Study the drawing (mm; zero at the part's minimum x, y, z) and answer. Coordinates: 2 decimals unless noted, no trailing zeros. Write each loop counter-clockwise with the first axis right and the second up, starting at its lowest first coordinate (ties: lowest second). Pieces come first, ordered by that corner, then holes. Notation, with made-up numbers: (-33, 66.5) -> (-9, 66.5) arc R17 cw to (-9, 93.5) -> close; hole circle Ø10 at (50.5, -9). An arc over 180 degrees is marked (long way). Write item = value, one per line. Start each with the question number.
1) Flat-ended cylindrical pins translate along their axes: pin 1 Ø8 at (y, z) = (230.5, 94.5) entering from +X; pin 2 Ø5 at (x, y) = (8, 4) entering from -Z; pin 3 Ø6.5 at (x, z) = (14.5, 8.5) entering from +Y. Find the tip coordinate at first contact, or state that the pin passes through.
2) Section C-C (x = 8.5) is taken. Determine the outline of the cut face in (y, z) (1 decimal).
3) For a pull along Z with two mould halves and no side action, classify the marked faces 1, 2, 3 and 4 as released by +Z, released by -Z, zero draft, split by the parting line, or undercut.
4) Section D-D (z = 141) is taken. Determine the outline of the cut face in (x, y), plus the area to 3 significant figures.
5) Section A-A (y = 261.5) is taken. Determine the outline of the cut face in (x, z).
6) Section B-B (z = 87) is taken. Determine the outline of the cut face in (x, y), plus the area to 3 significant figures.
7) Find the intervals of material crossed by line 1 along Y through (x, z) = (22.25, 101); line 2 along Z through (x, y) = (10.25, 279) (1 decimal); line 3 along Y through (x, z) = (17, 72.5), in increasing order. Write a range as from..to.
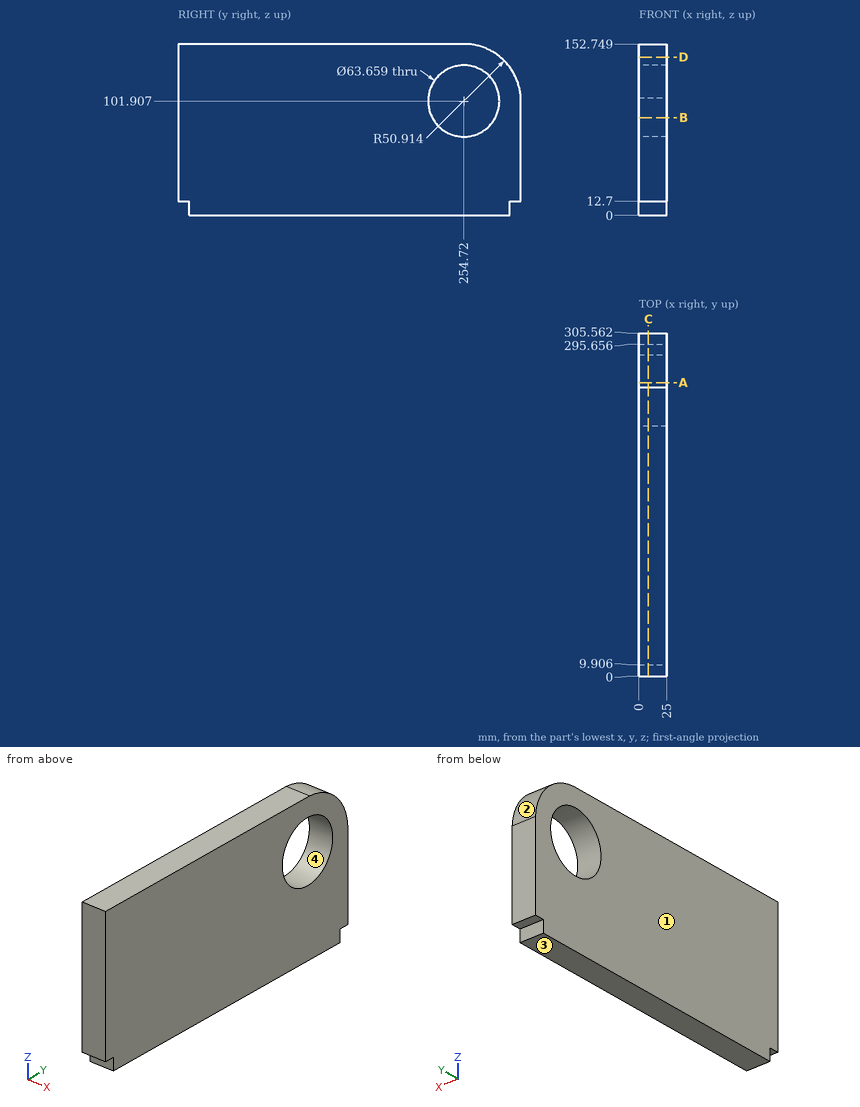
Answer key:
q1.pin_1 = through
q1.pin_2 = 12.7
q1.pin_3 = 295.66
q2.outline = (0, 12.7) -> (9.9, 12.7) -> (9.9, 0) -> (295.7, 0) -> (295.7, 12.7) -> (305.6, 12.7) -> (305.6, 104.6) arc R50.9 ccw to (257.4, 152.7) -> (0, 152.7) -> close; hole circle Ø63.7 at (254.7, 101.9)
q3.face_1 = zero draft
q3.face_2 = released by +Z
q3.face_3 = released by -Z
q3.face_4 = undercut
q4.outline = (0, 0) -> (25, 0) -> (25, 287.34) -> (0, 287.34) -> close
q4.area = 7,180 mm^2
q5.outline = (0, 0) -> (25, 0) -> (25, 70.81) -> (0, 70.81) -> close; (0, 133.01) -> (25, 133.01) -> (25, 152.37) -> (0, 152.37) -> close
q6.outline = (0, 0) -> (25, 0) -> (25, 226.6) -> (0, 226.6) -> close; (0, 282.84) -> (25, 282.84) -> (25, 305.56) -> (0, 305.56) -> close
q6.area = 6,230 mm^2
q7.line_1 = 0..222.9, 286.54..305.56
q7.line_2 = 0..81.3, 122.5..146.7
q7.line_3 = 0..242.54, 266.9..305.56
